Autodesk Inventor part; units mm, degrees
ref_plane "YZ Plane" through (0, 0, 0) normal (1, 0, 0) x (0, 1, 0)
ref_plane "XZ Plane" through (0, 0, 0) normal (0, 1, 0) x (-1, 0, 0)
ref_plane "XY Plane" through (0, 0, 0) normal (0, 0, 1) x (1, 0, 0)
sketch "스케치1" plane through (0, 0, 0) normal (0, 0, 1) x (1, 0, 0)
  circle A0 centre (0, 0) radius 22.5
  dimension "d0" = 45
extrude "돌출1" add sketch "스케치1" along normal blind 8
sketch "스케치2" plane through (0, 0, 8) normal (0, 0, 1) x (1, 0, 0)
  circle A0 centre (0, 0) radius 8
  dimension "d3" = 16
extrude "돌출2" cut sketch "스케치2" against normal up to surface (8 mm away)
sketch "스케치3" plane through (0, 0, 8) normal (0, 0, 1) x (1, 0, 0)
  line L0 (-0.15, -20.7995) -> (-0.15, -19.593)
  arc A0 (-0.15, -16.407) -> (-0.15, -19.593) centre (0, -18) ccw
  line L1 (-0.15, -16.407) -> (-0.15, -12.9991)
  arc A1 (0.15, -12.9991) -> (-0.15, -12.9991) centre (0, 0) ccw
  line L2 (0.15, -16.407) -> (0.15, -12.9991)
  arc A2 (0.15, -19.593) -> (0.15, -16.407) centre (0, -18) ccw
  line L3 (0.15, -20.7995) -> (0.15, -19.593)
  arc A3 (0.15, -20.7995) -> (-0.15, -20.7995) centre (0, 0) ccw
  circle A4 centre (12, 12) radius 1.6
  circle A5 centre (-18, 0) radius 1.6
  circle A6 centre (-12, 12) radius 1.6
  circle A7 centre (-12, -12) radius 1.6
  circle A8 centre (18, 0) radius 1.6
  circle A9 centre (12, -12) radius 1.6
  circle A10 centre (6, 18) radius 1
  circle A11 centre (-6, 18) radius 1
  circle A12 centre (-18, 6) radius 1
  circle A13 centre (-18, -6) radius 1
  circle A14 centre (-6, -18) radius 1
  circle A15 centre (6, -18) radius 1
  circle A16 centre (18, -6) radius 1
  circle A17 centre (18, 6) radius 1
  circle A18 centre (0, 18) radius 1.6
  circle A19 centre (0, 0) radius 12.5
  line L4 (-27, -21) -> (-21, -21)
  line L5 (-21, -21) -> (-21, -27)
  line L6 (25, -27) -> (27, -25)
  line L7 (27, -25) -> (27, 25)
  line L8 (27, 25) -> (25, 27)
  line L9 (25, 27) -> (-25, 27)
  line L10 (-25, 27) -> (-27, 25)
  line L11 (-27, 25) -> (-27, -25)
  line L12 (-27, -25) -> (-25, -27)
  line L13 (-25, -27) -> (25, -27)
  circle A20 centre (0, 0) radius 26.75
  circle A21 centre (24, -24) radius 1.6
  circle A22 centre (-24, -24) radius 1.6
  circle A23 centre (24, 24) radius 1.6
  circle A24 centre (-24, 24) radius 1.6
  circle A25 centre (0, -18) radius 1.6
  dimension "d6" = 3.2
extrude "돌출3" cut sketch "스케치3" against normal up to surface (8 mm away) contours A0 A25 A2 | A4 | A5 | A6 | A7 | A8 | A9 | A18
sketch "스케치4" plane through (0, 0, 8) normal (0, 0, 1) x (1, 0, 0)
  circle A0 centre (0, 18) radius 1.6
  circle A1 centre (-18, 0) radius 1.6
  circle A2 centre (-12, -12) radius 1.6
  circle A3 centre (12, 12) radius 1.6
  circle A4 centre (18, 0) radius 1.6
  circle A5 centre (0, -18) radius 1.6
  circle A6 centre (12, -12) radius 1.6
  circle A7 centre (-12, 12) radius 1.6
  circle A8 centre (0, 0) radius 8
  circle A9 centre (0, 0) radius 22.5
  circle A10 centre (-18, 0) radius 3
  circle A11 centre (-12, 12) radius 3
  circle A12 centre (0, 18) radius 1.6
  circle A13 centre (0, 18) radius 3
  circle A14 centre (12, 12) radius 1.6
  circle A15 centre (12, 12) radius 3
  circle A16 centre (18, 0) radius 3
  circle A17 centre (12, -12) radius 1.6
  circle A18 centre (12, -12) radius 3
  circle A19 centre (0, -18) radius 3
  circle A20 centre (-12, -12) radius 3
  dimension "d9" = 6
  dimension "d10" = 6
  dimension "d11" = 6
  dimension "d12" = 6
  dimension "d13" = 6
  dimension "d14" = 6
  dimension "d15" = 6
  dimension "d16" = 6
extrude "돌출4" cut sketch "스케치4" against normal blind 4 contours A10 | A11 | A13 | A15 | A16 | A18 | A19 | A20
sketch "스케치5" plane through (0, 0, 8) normal (0, 0, 1) x (1, 0, 0)
  line L0 (0, 0) -> (12.0104, 4.9749)
  line L1 (0, 0) -> (13, 0) construction
  circle A0 centre (12.0104, 4.9749) radius 1.25
  circle A1 centre (4.9749, 12.0104) radius 1.25
  circle A2 centre (-4.9749, 12.0104) radius 1.25
  circle A3 centre (-12.0104, 4.9749) radius 1.25
  circle A4 centre (-12.0104, -4.9749) radius 1.25
  circle A5 centre (-4.9749, -12.0104) radius 1.25
  circle A6 centre (4.9749, -12.0104) radius 1.25
  circle A7 centre (12.0104, -4.9749) radius 1.25
  dimension "d19" = 13
  dimension "d20" = 22.5
  dimension "d21" = 2.5
  dimension "d24" = 360
extrude "돌출5" cut sketch "스케치5" against normal up to surface (8 mm away)
equation "\"d4\" = d3"
properties part number "조인트1고관절축" material "알루미늄 6061"
Can you work these out from the model? Positions are in its coordinate system, mm. A direction names the side the tool comes from. Round coordinates to 2 decimals unless told otherwise and drop trailing zeros. Loops run counter-clockwise (first coordinate to the right, second up) from the corner with the lowest first, then second, coordinate; pieces in that order, holes last. Notation, with made-up numbers: (-3, 32.25) -> (4, 32.25) arc R9 ccw to (4, 40.25) -> close; hole circle Ø6 at (-26.75, 84). An arc over 180 degrees is marked (long way). One line per item, written item: value. Start each with the question number.
1. If we section it at B-B, the plane y = 0: Write out the boundary of the cut face in (x, z).
2. If we section it at A-A, the plane y = -18: Write out the boundary of the cut face in (x, z), then the cut area to 3 significant figures.
3. For pin 1 (1 mm diameter, centred on y = 13.5, z = 4.5, fed in from -X); pin 2 (1 mm diameter, centred on x = 1, z = 6, fed in from -Y), each with a flat end and sliding along its axis, tell me the tip position at first contact or that it passes through.
4. If we section it at D-D, the plane z = 1.5: Give the number of separate pieces and of enclosed holes in the cut face, then the cut area to 3 significant figures.
5. For faces 3 (the cylindrical face through (-0.65, -20.93, 6.03)), 4 (the cylindrical face through (-1.6, -18, 2)), which set-ups out of +Z, -Z, +X, -X, +Y, -Y let a thin tool reach every point of the face, with its end or its side?
6. If I drill on probe 1 along Y at (x, z) = (0, 6.25); probe 2 along X at (y, z) = (-13, 5); probe 3 along Y at (x, z) = (-14, 6.75), over which ranges is the centre line in solid material (lowest first)?
7. If we mould it in two halves opening along X, with no side actions, what happens to faces 1 (the flat face through (1.3, -19.3, 4)), 2 (the cylindrical face through (10.382, 19.961, 3.944))? For each: pulls with the +X half, pulls with the -X half, needs draft (parallel to the pull), parting line crosses it, or undercut.
Calculated:
1. outline: (-22.5, 0) -> (-19.6, 0) -> (-19.6, 4) -> (-21, 4) -> (-21, 8) -> (-22.5, 8) -> close; (-16.4, 0) -> (-8, 0) -> (-8, 8) -> (-15, 8) -> (-15, 4) -> (-16.4, 4) -> close; (8, 0) -> (16.4, 0) -> (16.4, 4) -> (15, 4) -> (15, 8) -> (8, 8) -> close; (19.6, 0) -> (22.5, 0) -> (22.5, 8) -> (21, 8) -> (21, 4) -> (19.6, 4) -> close
2. outline: (-13.5, 0) -> (-1.6, 0) -> (-1.6, 4) -> (-3, 4) -> (-3, 8) -> (-13.5, 8) -> close; (1.6, 0) -> (13.5, 0) -> (13.5, 8) -> (3, 8) -> (3, 4) -> (1.6, 4) -> close
2. area: 179 mm²
3. pin 1: stops at x = -18.36
3. pin 2: stops at y = -22.49
4. separate pieces: 1
4. enclosed holes: 17
4. area: 1,290 mm²
5. face 3: +Z
5. face 4: +Z, -Z
6. probe 1: y = -22.5 to -21, -15 to -8, 8 to 15, 21 to 22.5
6. probe 2: x = -18.36 to -14.83, -9.17 to -5.74, -4.21 to 4.21, 5.74 to 9.17, 14.83 to 18.36
6. probe 3: y = -17.61 to -14.24, -9.76 to 9.76, 14.24 to 17.61
7. face 1: undercut
7. face 2: parting line crosses it
